Verification items for the finished model (mm, model axes). Face numbers are marked on the shaded views. Give positions to 0.01 mm unless a question says otherwise; leave off trailing zeros. Answer in a Markdown table with one row per item. Add a question column.
Q1. Gauge pin test, flat ends, axial feed: P1, Ø4.5, axis at y = -3.5, z = 20, coming from the -X side; P2, Ø3, axis at x = 30, z = 30, coming from the -Y side; P3, Ø2, axis at x = 33, z = 8, coming from the -Y side; P4, Ø2, axis at x = -50.5, y = 3.5, coming from the +Z side. Record the tip position at first contact, or that the pin passes through.
Q2. Section check A-A on z = 30. Give the number of separate pieces and of enclosed holes in the cut face, and give its area (3 significant figures).
Q3. Material ranges on probe 1 along Z at (x, y) = (45, 0.5); probe 2 along Z at (x, y) = (-30, 6.25); probe 3 along X at (y, z) = (-4.5, 22.5), recorded low to high.
Q4. Release check for a two-part mould opening along Z. For the marked faces 1 and 2 record: pulls with the +Z half, pulls with the -Z half, needs draft (parallel to the pull), parting line crosses it, or undercut.
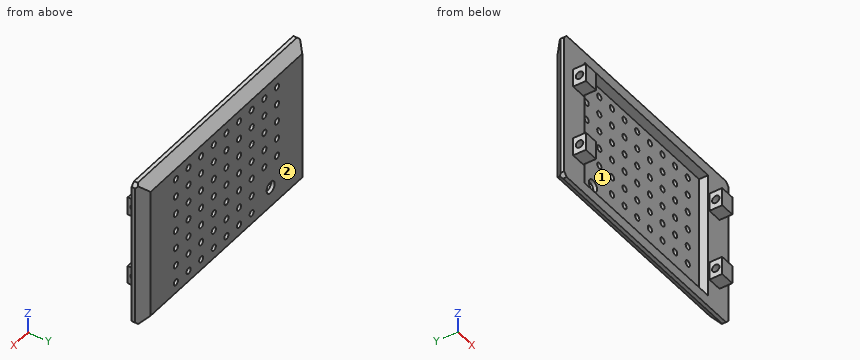
```python
from build123d import *

# Parameters (mm, degrees)
SKETCH1_W           = 130
SKETCH1_H           = 82
BOSS_EXTRUDE1_DEPTH = 2
SKETCH3_W           = 120
SKETCH3_H           = 72
SKETCH2_W           = 130
SKETCH2_H           = 82
CHAMFER2_SIZE       = 2
SKETCH4_W           = 8
SKETCH4_H           = 10
BOSS_EXTRUDE2_DEPTH = 7
SKETCH5_R           = 2.05
CUT_EXTRUDE1_DEPTH  = 123.9000001
SKETCH6_W           = 97.8
SKETCH6_H           = 70
CUT_EXTRUDE2_DEPTH  = 5
SKETCH7_R           = 1.65
CUT_EXTRUDE3_DEPTH  = 3.0000001
SKETCH8_R           = 3.2
CUT_EXTRUDE4_DEPTH  = 15
SKETCH9_R           = 1.65
BOSS_EXTRUDE3_DEPTH = 2


with BuildPart() as part:
    # Sketch1 → Boss-Extrude1 (new body)
    with BuildSketch(Plane(origin=(0, 0, 0), x_dir=(1, 0, 0), z_dir=(0, 1, 0))):
        Rectangle(SKETCH1_W, SKETCH1_H)
    extrude(amount=BOSS_EXTRUDE1_DEPTH)

    # Sketch3 → Loft1 section 0
    with BuildSketch(Plane(origin=(0, 7, 0), x_dir=(1, 0, 0), z_dir=(0, 1, 0))):
        Rectangle(SKETCH3_W, SKETCH3_H)
    # Sketch2 → Loft1 section 1
    with BuildSketch(Plane(origin=(0, 2, 0), x_dir=(1, 0, 0), z_dir=(0, 1, 0))):
        Rectangle(SKETCH2_W, SKETCH2_H)
    loft()

    # Chamfer2
    chamfer2_edges = [part.edges().sort_by_distance(p)[0] for p in [
        (65, 1, 41),
        (-65, 1, 41),
        (-65, 1, -41),
        (65, 1, -41),
    ]]
    chamfer(chamfer2_edges, length=CHAMFER2_SIZE)

    # Sketch4 → Boss-Extrude2 (add)
    with BuildSketch(Plane.XZ):
        with Locations((-53.9, 20)):
            Rectangle(SKETCH4_W, SKETCH4_H)
        with Locations((-53.9, -20)):
            Rectangle(SKETCH4_W, SKETCH4_H)
        with Locations((53.9, -20)):
            Rectangle(SKETCH4_W, SKETCH4_H)
        with Locations((53.9, 20)):
            Rectangle(SKETCH4_W, SKETCH4_H)
    extrude(amount=BOSS_EXTRUDE2_DEPTH)

    # Sketch5 → Cut-Extrude1 (cut, through all)
    with BuildSketch(Plane.ZY.offset(57.9)):
        with Locations((-20, -3.5)):
            Circle(SKETCH5_R)
        with Locations((20, -3.5)):
            Circle(SKETCH5_R)
    extrude(amount=-CUT_EXTRUDE1_DEPTH, mode=Mode.SUBTRACT)

    # Sketch6 → Cut-Extrude2 (cut)
    with BuildSketch(Plane.XZ):
        Rectangle(SKETCH6_W, SKETCH6_H)
    extrude(amount=-CUT_EXTRUDE2_DEPTH, mode=Mode.SUBTRACT)

    # Sketch7 → Cut-Extrude3 (cut, through all)
    with BuildSketch(Plane.XZ.offset(-5)):
        Circle(SKETCH7_R)
        with Locations((10, 0)):
            Circle(SKETCH7_R)
        with Locations((20, 0)):
            Circle(SKETCH7_R)
        with Locations((30, 0)):
            Circle(SKETCH7_R)
        with Locations((40, 0)):
            Circle(SKETCH7_R)
        with Locations((10, 10)):
            Circle(SKETCH7_R)
        with Locations((20, 10)):
            Circle(SKETCH7_R)
        with Locations((30, 10)):
            Circle(SKETCH7_R)
        with Locations((40, 10)):
            Circle(SKETCH7_R)
        with Locations((10, 20)):
            Circle(SKETCH7_R)
        with Locations((20, 20)):
            Circle(SKETCH7_R)
        with Locations((30, 20)):
            Circle(SKETCH7_R)
        with Locations((40, 20)):
            Circle(SKETCH7_R)
        with Locations((10, 30)):
            Circle(SKETCH7_R)
        with Locations((20, 30)):
            Circle(SKETCH7_R)
        with Locations((30, 30)):
            Circle(SKETCH7_R)
        with Locations((40, 30)):
            Circle(SKETCH7_R)
        with Locations((0, 10)):
            Circle(SKETCH7_R)
        with Locations((0, 20)):
            Circle(SKETCH7_R)
        with Locations((0, 30)):
            Circle(SKETCH7_R)
        with Locations((-40, 30)):
            Circle(SKETCH7_R)
        with Locations((-30, 30)):
            Circle(SKETCH7_R)
        with Locations((-20, 30)):
            Circle(SKETCH7_R)
        with Locations((-10, 30)):
            Circle(SKETCH7_R)
        with Locations((-40, 20)):
            Circle(SKETCH7_R)
        with Locations((-30, 20)):
            Circle(SKETCH7_R)
        with Locations((-20, 20)):
            Circle(SKETCH7_R)
        with Locations((-10, 20)):
            Circle(SKETCH7_R)
        with Locations((-40, 10)):
            Circle(SKETCH7_R)
        with Locations((-30, 10)):
            Circle(SKETCH7_R)
        with Locations((-20, 10)):
            Circle(SKETCH7_R)
        with Locations((-10, 10)):
            Circle(SKETCH7_R)
        with Locations((-40, 0)):
            Circle(SKETCH7_R)
        with Locations((-30, 0)):
            Circle(SKETCH7_R)
        with Locations((-20, 0)):
            Circle(SKETCH7_R)
        with Locations((-10, 0)):
            Circle(SKETCH7_R)
        with Locations((-10, -10)):
            Circle(SKETCH7_R)
        with Locations((-20, -10)):
            Circle(SKETCH7_R)
        with Locations((-30, -10)):
            Circle(SKETCH7_R)
        with Locations((-40, -10)):
            Circle(SKETCH7_R)
        with Locations((-10, -20)):
            Circle(SKETCH7_R)
        with Locations((-20, -20)):
            Circle(SKETCH7_R)
        with Locations((-30, -20)):
            Circle(SKETCH7_R)
        with Locations((-40, -20)):
            Circle(SKETCH7_R)
        with Locations((-10, -30)):
            Circle(SKETCH7_R)
        with Locations((-20, -30)):
            Circle(SKETCH7_R)
        with Locations((-30, -30)):
            Circle(SKETCH7_R)
        with Locations((-40, -30)):
            Circle(SKETCH7_R)
        with Locations((0, -30)):
            Circle(SKETCH7_R)
        with Locations((0, -20)):
            Circle(SKETCH7_R)
        with Locations((0, -10)):
            Circle(SKETCH7_R)
        with Locations((40, -30)):
            Circle(SKETCH7_R)
        with Locations((30, -30)):
            Circle(SKETCH7_R)
        with Locations((20, -30)):
            Circle(SKETCH7_R)
        with Locations((10, -30)):
            Circle(SKETCH7_R)
        with Locations((40, -20)):
            Circle(SKETCH7_R)
        with Locations((30, -20)):
            Circle(SKETCH7_R)
        with Locations((20, -20)):
            Circle(SKETCH7_R)
        with Locations((10, -20)):
            Circle(SKETCH7_R)
        with Locations((40, -10)):
            Circle(SKETCH7_R)
        with Locations((30, -10)):
            Circle(SKETCH7_R)
        with Locations((20, -10)):
            Circle(SKETCH7_R)
        with Locations((10, -10)):
            Circle(SKETCH7_R)
    extrude(amount=-CUT_EXTRUDE3_DEPTH, mode=Mode.SUBTRACT)

    # Sketch8 → Cut-Extrude4 (cut, through all)
    with BuildSketch(Plane(origin=(0, 7, 0), x_dir=(1, 0, 0), z_dir=(0, 1, 0))):
        with Locations((-35, 25)):
            Circle(SKETCH8_R)
    extrude(amount=-CUT_EXTRUDE4_DEPTH, mode=Mode.SUBTRACT)

    # Sketch9 → Boss-Extrude3 (add)
    with BuildSketch(Plane(origin=(0, 7, 0), x_dir=(1, 0, 0), z_dir=(0, 1, 0))):
        with Locations((-30, 20)):
            Circle(SKETCH9_R)
        with Locations((-40, 20)):
            Circle(SKETCH9_R)
        with Locations((-40, 30)):
            Circle(SKETCH9_R)
        with Locations((-30, 30)):
            Circle(SKETCH9_R)
    extrude(amount=-BOSS_EXTRUDE3_DEPTH)


solid = part.part
```
Taken from the geometry:
| question | item | result |
|---|---|---|
| 1 | P1 | stops at x = -57.9 |
| 1 | P2 | passes through |
| 1 | P3 | stops at y = 5 |
| 1 | P4 | stops at z = 40.5 |
| 2 | separate pieces | 10 |
| 2 | enclosed holes | 0 |
| 2 | area | 337 mm² |
| 3 | probe 1 | z = -41 to -35, 35 to 41 |
| 3 | probe 2 | z = -36.75 to -11.65, -8.35 to -1.65, 1.65 to 8.35, 11.65 to 18.35, 21.65 to 28.35, 31.65 to 36.75 |
| 3 | probe 3 | x = -57.9 to -49.9, 49.9 to 57.9 |
| 4 | face 1 | undercut |
| 4 | face 2 | needs draft |
